Check sheet for the drawn part. Datum: minimum x, y, z corner. Units: mm. Coordinates: 2 decimals unless noted, no trailing zeros. Order: outer loops, then holes, each group sorted by start corner. A loop starts at its lowest first (then second) coordinate and runs counter-clockwise, first axis right, second up. Notation, with made-up numbers: (82.25, -39.5) - (97.25, -39.5) arc R29 ccw to (97.25, -14.5) - close; hole circle Ø10 at (63, 69). An arc over 180 degrees is marked (long way). Answer as CSV lines item,"result". Start each with the question number.
1. Go/stop test with flat-tipped pins: pin 1 (0.9 mm diameter, centred on x = 1.5, y = 1, fed in from -Z); pin 2 (0.9 mm diameter, centred on x = 2, z = 32.5, fed in from -Y); pin 3 (1.5 mm diameter, centred on x = 2, y = 2, fed in from +Z). Record where each tip stops, or that it passes through.
2. Material ranges on L1, parallel to Z at x = 1.7, y = 1.5; L2, parallel to Y at x = 0.5, z = 55; L3, parallel to Y at x = 0.8, z = 22, recorded low to high. Write a range as [from, to].
3. Section check B-B (y = 23.75). Record the cut outline in (x, z).
4. Section check D-D (z = 9). Record the cut outline in (x, y), and give its area (3 significant figures).
5. Section check C-C (z = 30). Record the cut outline in (x, y), and give its area (3 significant figures).
6. Section check A-A (x = 0.8). Record the cut outline in (y, z), and give its area (3 significant figures).
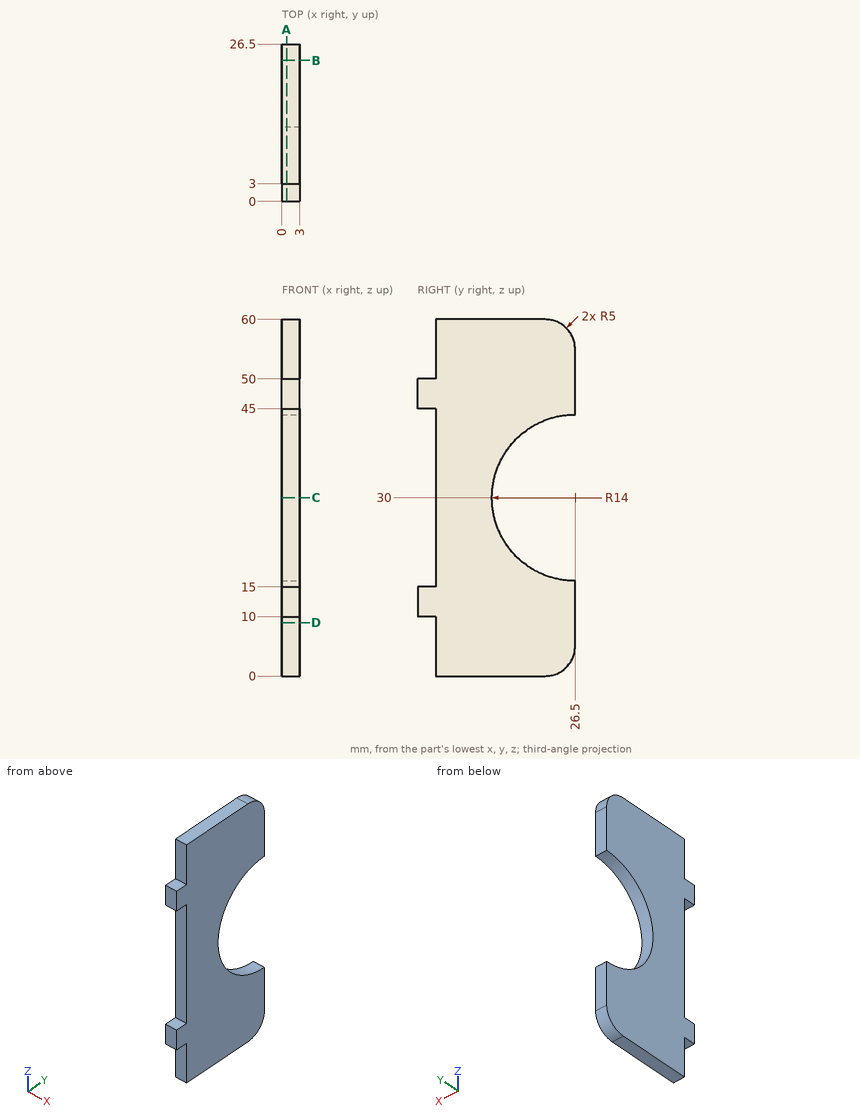
Evaluation:
1,pin 1,"stops at z = 10"
1,pin 2,"stops at y = 3"
1,pin 3,"stops at z = 50"
2,L1,"z = [10, 15], [45, 50]"
2,L2,"y = [3, 26.5]"
2,L3,"y = [3, 15.01]"
3,outline,"(0, 0.53) - (3, 0.53) - (3, 16.27) - (0, 16.27) - close; (0, 43.73) - (3, 43.73) - (3, 59.47) - (0, 59.47) - close"
4,outline,"(0, 3) - (3, 3) - (3, 26.5) - (0, 26.5) - close"
4,area,"70.5 mm²"
5,outline,"(0, 3) - (3, 3) - (3, 12.5) - (0, 12.5) - close"
5,area,"28.5 mm²"
6,outline,"(0, 10) - (3, 10) - (3, 0) - (21.5, 0) arc R5 ccw to (26.5, 5) - (26.5, 16) arc R14 cw to (26.5, 44) - (26.5, 55) arc R5 ccw to (21.5, 60) - (3, 60) - (3, 50) - (0, 50) - (0, 45) - (3, 45) - (3, 15) - (0, 15) - close"
6,area,"1,120 mm²"
